Drawing for the job (mm, zero at the part's lowest x, y, z). A direction names the side the tool comes from. Coordinates: 2 decimals unless noted, no trailing zeros. Order: outer loops, then holes, each group sorted by start corner. A loop starts at its lowest first (then second) coordinate and runs counter-clockwise, first axis right, second up.
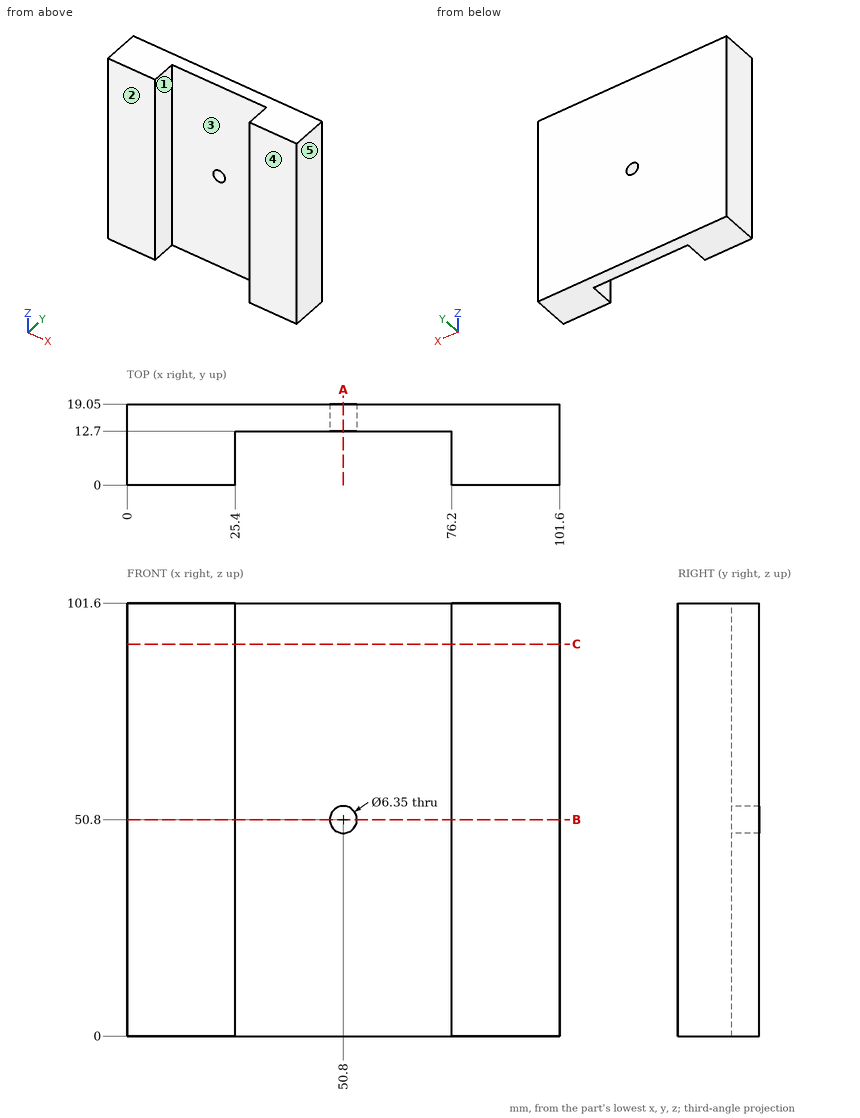
1) Two-plate mould, pull along X, no slides. Class the marked faces 3, 4 and 5: released by +X, released by -X, zero draft, split by the parting line, or undercut.
2) Slice it at A-A (x = 50.8). List the corners of the cut face in (y, z) (3 decimals), plus the area to 3 significant figures.
3) Pin check, flat tips, straight feed: P1, Ø5, axis at x = 50.8, z = 50.8, coming from the +Y side; P2, Ø6, axis at x = 44.5, z = 14.5, coming from the -Y side. Stop position of each tip, or through.
4) Slice it at C-C (z = 92). List the corners of the cut face in (x, y).
5) Which spindle directions (+Z, -Z, +X, -X, +Y, -Y) get a long thin tool onto all of the face, cutting with end or side? Do the marked faces 1 and 2. Say none if no direction does.
6) Drill centre lines: probe 1 along Z at (x, y) = (50.8, 16.75) (3 decimals); probe 2 along X at (y, z) = (1.25, 38); probe 3 along Y at (x, z) = (60, 17.5). Where is each one in solid material? Low to high.
7) Slice it at B-B (z = 50.8). List the corners of the cut face in (x, y) (3 decimals).
Worked out:
1. face 3: undercut
1. face 4: zero draft
1. face 5: released by +X
2. outline: (12.7, 0) - (19.05, 0) - (19.05, 47.625) - (12.7, 47.625) - close; (12.7, 53.975) - (19.05, 53.975) - (19.05, 101.6) - (12.7, 101.6) - close
2. area: 605 mm2
3. P1: passes through
3. P2: stops at y = 12.7
4. outline: (0, 0) - (25.4, 0) - (25.4, 12.7) - (76.2, 12.7) - (76.2, 0) - (101.6, 0) - (101.6, 19.05) - (0, 19.05) - close
5. face 1: +Z, -Z, -Y
5. face 2: +Z, -Z, +X, -X, -Y
6. probe 1: z = 0 to 47.625, 53.975 to 101.6
6. probe 2: x = 0 to 25.4, 76.2 to 101.6
6. probe 3: y = 12.7 to 19.05
7. outline: (0, 0) - (25.4, 0) - (25.4, 12.7) - (47.625, 12.7) - (47.625, 19.05) - (0, 19.05) - close; (53.975, 12.7) - (76.2, 12.7) - (76.2, 0) - (101.6, 0) - (101.6, 19.05) - (53.975, 19.05) - close
